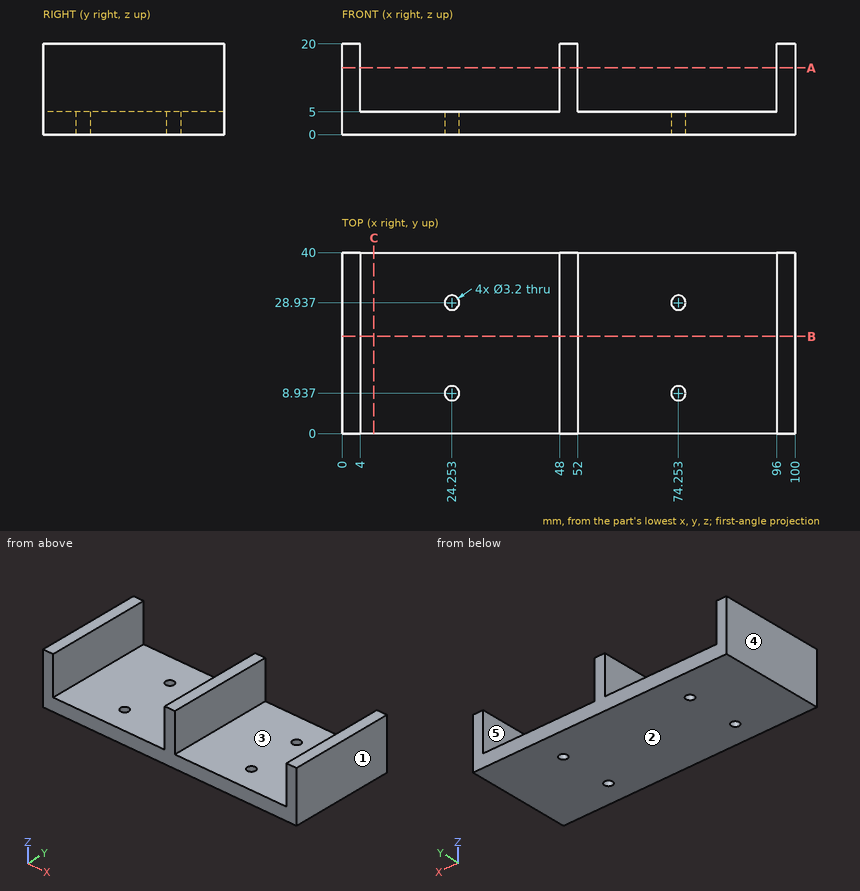
Design review of the part shown in the three views and the two pictorial views. Dimensions are in mm from the part's minimum x, y and z. A direction names the side the tool comes from. Round coordinates to 2 decimals unless told otherwise and drop trailing zeros. Loops run counter-clockwise (first coordinate to the right, second up) from the corner with the lowest first, then second, coordinate; pieces in that order, holes last. Notation, with made-up numbers: M -12,-34.75 L 40,-34.75 A24 ccw 40,-13.75 Z; hole C -23,35 d1. An arc over 180 degrees is marked long. Answer as a JSON object with one key per item and string values.
Item 1: Machinability: for the marked faces 4 and 5, which of the approach directions +Z, -Z, +X, -X, +Y, -Y give a long, thin tool a straight path to every point of the face, cutting with its end or side? Answer none if there is none.
Answer sheet:
{"face 4": "+Z, -Z, -X, +Y, -Y", "face 5": "+Z, +Y, -Y"}
Item 2: The part is to be moulded in two halves that separate along X. For the marked faces 1, 2 and 3, say which applies: pulls with the +X half, pulls with the -X half, needs draft (parallel to the pull), parting line crosses it, or undercut.
Answer sheet:
{"face 1": "pulls with the +X half", "face 2": "needs draft", "face 3": "undercut"}
Item 3: Wall thickness on L1, parallel to X at y = 9, z = 12.25; L2, parallel to Z at x = 71.5, y = 20.5: over which ranges is each line inside the solid? List them lowest first. Write a range as from..to.
Answer sheet:
{"L1": "x = 0..4, 48..52, 96..100", "L2": "z = 0..5"}
Item 4: We need section B-B on y = 21.5. Give the boundary of the cut face in (x, z).
Answer sheet:
{"outline": "M 0,0 L 100,0 L 100,20 L 96,20 L 96,5 L 52,5 L 52,20 L 48,20 L 48,5 L 4,5 L 4,20 L 0,20 Z"}
Item 5: Clearance check with flat-ended pins moving along their axes: P1, Ø12, axis at y = 14.5, z = 10.5, coming from the -X side; P2, Ø2.5, axis at x = 24.25, y = 28.94, coming from the +Z side; P3, Ø6, axis at x = 87.5, y = 26.5, coming from the +Z side. State where each tip first meets the part, or that it passes through.
Answer sheet:
{"P1": "stops at x = 0", "P2": "passes through", "P3": "stops at z = 5"}
Item 6: We need section A-A on z = 14.75. Give the boundary of the cut face in (x, y).
Answer sheet:
{"outline": "M 0,0 L 4,0 L 4,40 L 0,40 Z; M 48,0 L 52,0 L 52,40 L 48,40 Z; M 96,0 L 100,0 L 100,40 L 96,40 Z"}
Item 7: We need section C-C on x = 7. Give the boundary of the cut face in (y, z).
Answer sheet:
{"outline": "M 0,0 L 40,0 L 40,5 L 0,5 Z"}
